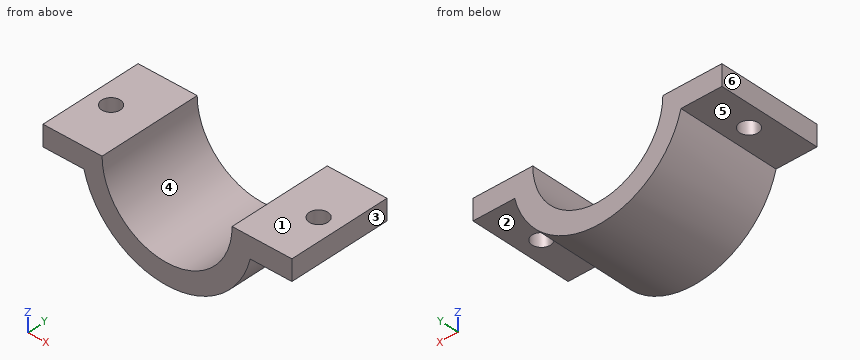
from build123d import *

# Parameters (mm, degrees)
BOSS_EXTRUDE1_DEPTH = 25.4
SKETCH2_R           = 2.286
CUT_EXTRUDE1_DEPTH  = 6.08


with BuildPart() as part:
    # Sketch1 → Boss-Extrude1 (new body)
    with BuildSketch(Plane(origin=(0, 0, 0), x_dir=(1, 0, 0), z_dir=(0, 1, 0))):
        with BuildLine():
            Line((-26.035, 0), (-16.002, 0))
            ThreePointArc((-16.002, 0), (0, 16.002), (16.002, 0))
            Line((16.002, 0), (26.035, 0))
            Line((26.035, 0), (30.716650549, 0))
            Line((30.716650549, 0), (30.716650549, 5.08))
            Line((30.716650549, 5.08), (26.035, 5.08))
            Line((26.035, 5.08), (20.460799691, 5.08))
            ThreePointArc((20.460799691, 5.08), (0, 21.082), (-20.460799691, 5.08))
            Line((-20.460799691, 5.08), (-26.035, 5.08))
            Line((-26.035, 5.08), (-30.543065264, 5.08))
            Line((-30.543065264, 5.08), (-30.543065264, 0))
            Line((-30.543065264, 0), (-26.035, 0))
        make_face()
    extrude(amount=BOSS_EXTRUDE1_DEPTH)

    # Sketch2 → Cut-Extrude1 (cut, through all)
    with BuildSketch(Plane(origin=(0, 0, -5.08), x_dir=(-1, 0, 0), z_dir=(0, 0, -1))):
        with Locations((-25.58872512, 12.7)):
            Circle(SKETCH2_R)
        with Locations((25.501932478, 12.7)):
            Circle(SKETCH2_R)
    extrude(amount=-CUT_EXTRUDE1_DEPTH, mode=Mode.SUBTRACT)


solid = part.part
The listing builds one solid part. Answer for the finished solid, in the listing's coordinates (mm). Face numbers are marked on the shaded views. A direction names the side the tool comes from. Coordinates: 2 decimals unless noted, no trailing zeros. Loops run counter-clockwise (first coordinate to the right, second up) from the corner with the lowest first, then second, coordinate; pieces in that order, holes last. Notation, with made-up numbers: M 35.25,69.5 L 91.25,69.5 A7 ccw 91.25,77.5 Z; hole C -7,54 d6. An arc over 180 degrees is marked long. Answer in a Markdown table with one row per item.
1) Given pin 1 (8 mm diameter, centred on x = 26.5, y = 13, fed in from -Z); pin 2 (3 mm diameter, centred on y = 13, z = -9.5, fed in from +X); pin 3 (1.5 mm diameter, centred on x = -11.5, y = 20, fed in from +Z); pin 4 (4 mm diameter, centred on x = -25.5, y = 12.7, fed in from +Z), each flat-ended and moving along its own axis, determine where each tip first touches the part or whether it passes through.
Answers below:
| item | result |
|---|---|
| pin 1 | z = -5.08 |
| pin 2 | x = 19.51 |
| pin 3 | z = -10.3 |
| pin 4 | through |
2) Determine the mould class of the marked faces 3, 4, 5 and 6 for opening direction X: released by +X, released by -X, zero draft, split by the parting line, or undercut.
Answers below:
| item | result |
|---|---|
| face 3 | released by +X |
| face 4 | undercut |
| face 5 | zero draft |
| face 6 | released by -X |
3) Find section B-B (z = -12.75). Determine the outline of the cut face in (x, y).
Answers below:
| item | result |
|---|---|
| outline | M -16.79,0 L -9.67,0 L -9.67,25.4 L -16.79,25.4 Z; M 9.67,0 L 16.79,0 L 16.79,25.4 L 9.67,25.4 Z |
4) Find section D-D (y = 4). Determine the outline of the cut face in (x, z), then the cut area to 3 significant figures.
Answers below:
| item | result |
|---|---|
| outline | M -30.54,-5.08 L -20.46,-5.08 A21.08 ccw 20.46,-5.08 L 30.72,-5.08 L 30.72,0 L 16,0 A16 cw -16,0 L -30.54,0 Z |
| area | 395 mm^2 |
5) Find section A-A (y = 12.7). Determine the outline of the cut face in (x, z).
Answers below:
| item | result |
|---|---|
| outline | M -30.54,-5.08 L -27.79,-5.08 L -27.79,0 L -30.54,0 Z; M -23.22,-5.08 L -20.46,-5.08 A21.08 ccw 20.46,-5.08 L 23.3,-5.08 L 23.3,0 L 16,0 A16 cw -16,0 L -23.22,0 Z; M 27.87,-5.08 L 30.72,-5.08 L 30.72,0 L 27.87,0 Z |
6) Which of the six approach directions +Z, -Z, +X, -X, +Y, -Y give full straight-line access (tool end or side, diameter ignored) to the marked faces 1 and 2?
Answers below:
| item | result |
|---|---|
| face 1 | +Z, +X, -X, +Y, -Y |
| face 2 | -Z, +X, +Y, -Y |
7) Find the intervals of material crossed by probe 1 along Z at (x, y) = (-26.5, 22.75); probe 2 along X at (y, z) = (8, -11.5); probe 3 along X at (y, z) = (23.25, -4.5), in increasing order.
Answers below:
| item | result |
|---|---|
| probe 1 | -5.08 to 0 |
| probe 2 | -17.67 to -11.13, 11.13 to 17.67 |
| probe 3 | -30.54 to -15.36, 15.36 to 30.72 |
8) Find section C-C (x = 26.5). Determine the outline of the cut face in (y, z), then the cut area to 3 significant figures.
Answers below:
| item | result |
|---|---|
| outline | M 0,-5.08 L 10.6,-5.08 L 10.6,0 L 0,0 Z; M 14.8,-5.08 L 25.4,-5.08 L 25.4,0 L 14.8,0 Z |
| area | 108 mm^2 |
